Geometry check sheet. Reference: the model listing, model coordinates, mm. Give positions to 0.01 mm unless a question says otherwise; leave off trailing zeros. Write each loop counter-clockwise with the first axis right and the second up, starting at its lowest first coordinate (ties: lowest second). Pieces come first, ordered by that corner, then holes.
(1) Mould release check, pull along X, two halves, no side actions. Record for faces 1 (the flat face through (38, 101.6, 3)), 2 (the flat face through (76.2, 25, 3)), 3 (the cylindrical face through (60.25, 12.56, 3.13)), 4 (the flat face through (0, 26, 3)): +X half, -X half, draft (parallel to the pull), parting line (faces both ways), or undercut.
(2) Thickness scan on line 1 along Y through (x, z) = (12.7, 2.25); line 2 along Y through (x, z) = (38.1, 4.75); line 3 along Y through (x, z) = (37.5, 4.5). Record the ranges inside material, lowest first.
(3) Cross-section at B-B (y = 38.1). Record the boundary of the cut face in (x, z).
(4) Depth check by flat-ended pin: P1, Ø3, axis at y = 66.5, z = 4.5, coming from the +X side; P2, Ø2, axis at y = 67.5, z = 5, coming from the +X side. Enter the tip coordinate at first touch or a pass-through.
(5) Cross-section at A-A (x = 63.5). Record the boundary of the cut face in (y, z).
(6) Cross-section at D-D (z = 3.5). Count the separate pieces of the cut face and the enclosed holes in it, and give its area (3 significant figures).
(7) Cross-section at C-C (y = 63.5). Record the boundary of the cut face in (x, z).
Autodesk Inventor part; units mm, degrees
ref_plane "YZ Plane" through (0, 0, 0) normal (1, 0, 0) x (0, 1, 0)
ref_plane "XZ Plane" through (0, 0, 0) normal (0, 1, 0) x (-1, 0, 0)
ref_plane "XY Plane" through (0, 0, 0) normal (0, 0, 1) x (1, 0, 0)
sketch "Sketch1" plane through (0, 0, 0) normal (0, 0, 1) x (1, 0, 0)
  line L0 (0, 0) -> (76.2, 0)
  line L1 (76.2, 0) -> (76.2, 50.8)
  line L2 (0, 50.8) -> (0, 0)
  line L3 (0, 0) -> (50.8, 0)
  line L4 (50.8, 101.6) -> (25.4, 101.6)
  line L5 (0, 50.8) -> (0, 0)
  line L6 (25.4, 101.6) -> (0, 50.8)
  line L7 (50.8, 101.6) -> (76.2, 50.8)
  line L8 (76.2, 50.8) -> (0, 50.8) construction
  circle A0 centre (12.7, 12.7) radius 3.2512
  circle A1 centre (12.7, 38.1) radius 3.2512
  circle A2 centre (38.1, 12.7) radius 3.2512
  circle A3 centre (38.1, 38.1) radius 3.2512
  circle A4 centre (63.5, 12.7) radius 3.2512
  circle A5 centre (63.5, 38.1) radius 3.2512
  circle A6 centre (38.1, 63.5) radius 3.2512
  circle A7 centre (38.1, 88.9) radius 3.2512
  dimension "d10" = 50.8
  dimension "d13" = 76.2
  dimension "d14" = 25.4
  dimension "d15" = 25.4
  dimension "d16" = 50.8
  dimension "d17" = 6.5024
  dimension "d18" = 12.7
  dimension "d19" = 12.7
  dimension "d22" = 25.4
  dimension "d25" = 25.4
  dimension "d30" = 25.4
extrude "Extrusion1" add sketch "Sketch1" along normal blind 6.35
properties part number "1x3 t plate"
Reply:
1. face 1: draft
1. face 2: +X half
1. face 3: undercut
1. face 4: -X half
2. line 1: y = 0 to 9.45, 15.95 to 34.85, 41.35 to 76.2
2. line 2: y = 0 to 9.45, 15.95 to 34.85, 41.35 to 60.25, 66.75 to 85.65, 92.15 to 101.6
2. line 3: y = 0 to 9.5, 15.9 to 34.9, 41.3 to 60.3, 66.7 to 85.7, 92.1 to 101.6
3. outline: (0, 0) - (9.45, 0) - (9.45, 6.35) - (0, 6.35) - close; (15.95, 0) - (34.85, 0) - (34.85, 6.35) - (15.95, 6.35) - close; (41.35, 0) - (60.25, 0) - (60.25, 6.35) - (41.35, 6.35) - close; (66.75, 0) - (76.2, 0) - (76.2, 6.35) - (66.75, 6.35) - close
4. P1: stops at x = 69.1
4. P2: stops at x = 68.35
5. outline: (0, 0) - (9.45, 0) - (9.45, 6.35) - (0, 6.35) - close; (15.95, 0) - (34.85, 0) - (34.85, 6.35) - (15.95, 6.35) - close; (41.35, 0) - (76.2, 0) - (76.2, 6.35) - (41.35, 6.35) - close
6. separate pieces: 1
6. enclosed holes: 8
6. area: 6,190 mm2
7. outline: (6.35, 0) - (34.85, 0) - (34.85, 6.35) - (6.35, 6.35) - close; (41.35, 0) - (69.85, 0) - (69.85, 6.35) - (41.35, 6.35) - close
